```python
from build123d import *

# Parameters (mm, degrees)
F0_W     = 94.5642
F0_H     = 79.9338
F1_DEPTH = 4.1148
F2_W     = 22.5171
F2_H     = 2.54
F2_W_2   = 49.53
F2_W_3   = 1.4234517733
F3_DEPTH = 13.97
F4_W     = 32.766
F4_H     = 15.24
F5_DEPTH = 2.286
F7_W     = 49.53
F7_H     = 5.969
F7_H_2   = 2.54
F7_H_3   = 6.7818
F8_DEPTH = 9.779
F6_R     = 1.524
F9_DEPTH = 25.4


with BuildPart() as f1:
    # F0 (on Top) → F1 (new body)
    with BuildSketch(Plane.XY):
        Rectangle(F0_W, F0_H)
        with BuildLine():
            Line((-40.3606, 3.3655), (-33.5026, 3.3655))
            ThreePointArc((-33.5026, 3.3655), (-30.1371, 0), (-33.5026, -3.3655))
            Line((-33.5026, -3.3655), (-40.3606, -3.3655))
            ThreePointArc((-40.3606, -3.3655), (-43.7261, 0), (-40.3606, 3.3655))
        make_face(mode=Mode.SUBTRACT)
        with BuildLine():
            Line((33.5026, 3.3655), (40.3606, 3.3655))
            ThreePointArc((40.3606, 3.3655), (43.7134059906, -0.0063380302), (40.3479, -3.3655))
            Line((40.3479, -3.3655), (33.4899, -3.3655))
            ThreePointArc((33.4899, -3.3655), (30.1243940094, 0.0063619924), (33.5026, 3.3655))
        make_face(mode=Mode.SUBTRACT)
    extrude(amount=F1_DEPTH)

    # F2 (on face) → F3 (join, symmetric)
    with BuildSketch(Plane.XY.offset(4.1148)):
        with Locations((36.02355, -38.6969)):
            Rectangle(F2_W, F2_H)
        with Locations((-36.02355, 38.6969)):
            Rectangle(F2_W, F2_H)
        with Locations((-36.02355, -38.6969)):
            Rectangle(F2_W, F2_H)
        with Locations((0, 38.6969)):
            Rectangle(F2_W_2, F2_H)
        with Locations((36.02355, 30.1879)):
            Rectangle(F2_W, F2_H)
        with Locations((36.02355, 21.6789)):
            Rectangle(F2_W, F2_H)
        with Locations((36.02355, 13.1699)):
            Rectangle(F2_W, F2_H)
        with Locations((36.02355, -13.1699)):
            Rectangle(F2_W, F2_H)
        with Locations((36.02355, -21.6789)):
            Rectangle(F2_W, F2_H)
        with Locations((36.02355, -30.1879)):
            Rectangle(F2_W, F2_H)
        with Locations((0, -38.6969)):
            Rectangle(F2_W_2, F2_H)
        with Locations((-36.02355, 30.1879)):
            Rectangle(F2_W, F2_H)
        with Locations((-36.02355, 21.6789)):
            Rectangle(F2_W, F2_H)
        with Locations((-36.02355, 13.1699)):
            Rectangle(F2_W, F2_H)
        with Locations((-36.02355, -13.1699)):
            Rectangle(F2_W, F2_H)
        with Locations((-36.02355, -21.6789)):
            Rectangle(F2_W, F2_H)
        with Locations((-36.02355, -30.1879)):
            Rectangle(F2_W, F2_H)
        with Locations((0, 30.1879)):
            Rectangle(F2_W_2, F2_H)
        with Locations((0, 21.6789)):
            Rectangle(F2_W_2, F2_H)
        with Locations((0, 13.1699)):
            Rectangle(F2_W_2, F2_H)
        with Locations((0, -13.1699)):
            Rectangle(F2_W_2, F2_H)
        with Locations((0, -21.6789)):
            Rectangle(F2_W_2, F2_H)
        with Locations((0, -30.1879)):
            Rectangle(F2_W_2, F2_H)
        with Locations((0, 4.6609)):
            Rectangle(F2_W_2, F2_H)
        with Locations((0, -4.6609)):
            Rectangle(F2_W_2, F2_H)
        with Locations((47.9938258867, 38.6969)):
            Rectangle(F2_W_3, F2_H)
        with Locations((36.02355, 38.6969)):
            Rectangle(F2_W, F2_H)
    extrude(amount=F3_DEPTH, both=True)

    # F4 (on face) → F5 (join)
    with BuildSketch(Plane(origin=(0, 39.9669, 0), x_dir=(-1, 0, 0), z_dir=(0, 1, 0))):
        Rectangle(F4_W, F4_H)
    extrude(amount=F5_DEPTH)

    # F7 (on face) → F8 (join)
    with BuildSketch(Plane(origin=(0, 0, 0), x_dir=(1, 0, 0), z_dir=(0, 0, -1))):
        with Locations((0, 8.9154)):
            Rectangle(F7_W, F7_H)
        with Locations((0, 4.6609)):
            Rectangle(F7_W, F7_H_2)
        Rectangle(F7_W, F7_H_3)
        with Locations((0, -4.6609)):
            Rectangle(F7_W, F7_H_2)
        with Locations((0, -8.9154)):
            Rectangle(F7_W, F7_H)
    extrude(amount=F8_DEPTH)

    # F6 (on face) → F9 (join)
    with BuildSketch(Plane(origin=(0, 42.2529, 0), x_dir=(-1, 0, 0), z_dir=(0, 1, 0))):
        with Locations((-8.1915, 3.81)):
            Circle(F6_R)
        with Locations((8.1915, 3.81)):
            Circle(F6_R)
        with Locations((4.09575, 0)):
            Circle(F6_R)
        with Locations((-4.09575, 0)):
            Circle(F6_R)
        with Locations((8.1915, -3.7334442604)):
            Circle(F6_R)
        with Locations((-8.1915, -3.81)):
            Circle(F6_R)
        with Locations((0, 3.81)):
            Circle(F6_R)
        with Locations((0, -3.81)):
            Circle(F6_R)
    extrude(amount=F9_DEPTH)


solid = f1.part
```
Can you work these out from the model? Positions are in its coordinate system, mm. A direction names the side the tool comes from. Round coordinates to 2 decimals unless told otherwise and drop trailing zeros. Loops run counter-clockwise (first coordinate to the right, second up) from the corner with the lowest first, then second, coordinate; pieces in that order, holes last. Notation, with made-up numbers: M 41,87 L 48,87 A18 cw 48,117 Z; hole C 24,44.25 d4. An arc over 180 degrees is marked long. Answer as a JSON object with one key per item and string values. Group by question number.
Q1. Imagine slicing it at B-B, the plane z = 12.5. Count the separate pieces of the cut face and the enclosed holes in it, then the cut area to 3 significant figures.
Q2. We'd pull the mould along Y, two halves only. Please class faces 1 (the flat face through (-24.765, 5, 11)), 2 (the flat face through (-8, 67.653, 4)), 3 (the flat face through (-1, 30, -9.855)), 4 (the flat face through (-1, -22.949, -5)): +Y half, -Y half, draft (parallel to the pull), parting line (faces both ways), or undercut.
Q3. Imagine slicing it at A-A, the plane y = 0. Please give me the cut outline in (x, z) (3 decimals).
Q4. On a 3-axis mill with a long thin cutter (end or side, diameter ignored), from which of +Z, -Z, +X, -X, +Y, -Y can I reach the whole of each face in a straight line? I mean faces 5 (the flat face through (-16.383, 41, 0)), 6 (the flat face through (-1, -34, 0)), 7 (the flat face through (37, 3.366, 2)), 8 (the flat face through (1, -37.427, 11)), 9 (the flat face through (-24.765, 0, -5)). Say none if no direction works.
Q5. Will these pins go through, and if not, where does the flat tip stop? pin 1 (4.5 mm diameter, centred on x = 38, z = 1.5, fed in from +Y); pin 2 (1.8 mm diameter, centred on x = -9.5, y = -34, fed in from +Z); pin 3 (0.7 mm diameter, centred on x = 8, y = 41.5, fed in from +Z).
Q6. Imagine slicing it at D-D, the plane y = -33. Please give me the cut outline in (x, z), then the cut area to 3 significant figures.
Q7. Imagine slicing it at C-C, the plane y = 59.5. Please give me the cut outline in (x, z), then the cut area to 3 significant figures.
Q8. Please list where these lines run through material, in increasing order: L1, parallel to Y at x = -38.5, z = 1; L2, parallel to X at y = 61, z = 2.75; L3, parallel to Y at x = 27.5, z = 0.5.
Findings:
{
 "1": {"separate pieces": "10", "enclosed holes": "0", "area": "2,180 mm2"},
 "2": {"face 1": "undercut", "face 2": "+Y half", "face 3": "draft", "face 4": "undercut"},
 "3": {"outline": "M -47.282,0 L -43.726,0 L -43.726,4.115 L -47.282,4.115 Z; M -30.137,0 L -24.765,0 L -24.765,-9.779 L 24.765,-9.779 L 24.765,0 L 30.124,0 L 30.124,4.115 L -30.137,4.115 Z; M 43.713,0 L 47.282,0 L 47.282,4.115 L 43.713,4.115 Z"},
 "4": {"face 5": "+Z, -Z, -X, +Y", "face 6": "-Z, +X, -X", "face 7": "+Z, -Z", "face 8": "+Z, +X, -X", "face 9": "-Z, -X"},
 "5": {"pin 1": "stops at y = 39.97", "pin 2": "stops at z = 4.11", "pin 3": "stops at z = 7.62"},
 "6": {"outline": "M -47.28,0 L 47.28,0 L 47.28,4.11 L -47.28,4.11 Z", "area": "389 mm2"},
 "7": {"outline": "C -8.19,-3.73 d3.05; C -8.19,3.81 d3.05; C -4.1,0 d3.05; C 0,-3.81 d3.05; C 0,3.81 d3.05; C 4.1,0 d3.05; C 8.19,-3.81 d3.05; C 8.19,3.81 d3.05", "area": "58.4 mm2"},
 "8": {"L1": "y = -39.97 to -3.37, 3.37 to 39.97", "L2": "x = -9.29 to -7.1, -1.09 to 1.09, 7.1 to 9.29", "L3": "y = -39.97 to 39.97"}
}
